Can you work these out from the model? Positions are in its coordinate system, mm. Face numbers are marked on the shaded views. Round coordinates to 2 decimals unless told otherwise and drop trailing zeros. Loops run counter-clockwise (first coordinate to the right, second up) from the corner with the lowest first, then second, coordinate; pieces in that order, holes last.
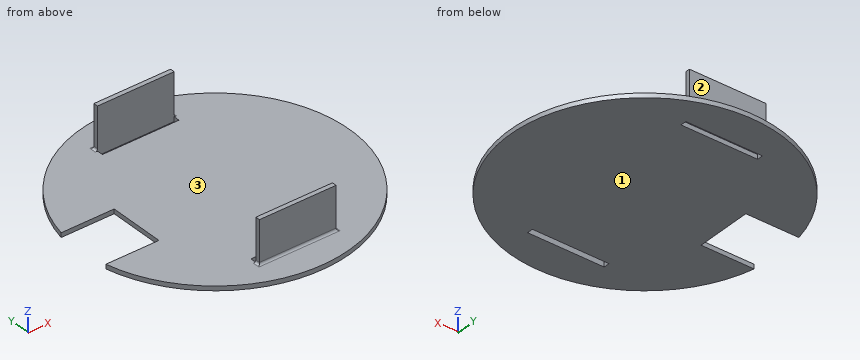
```python
from build123d import *

# Parameters (mm, degrees)
CROQUIS1_W              = 34.2
CROQUIS1_H              = 2.7
SALIENTE_EXTRUIR1_DEPTH = 2
CROQUIS2_W              = 34.2
CROQUIS2_H              = 2
SALIENTE_EXTRUIR2_DEPTH = 19
REDONDEO1_R             = 1


with BuildPart() as part:
    # Croquis1 → Saliente-Extruir1 (new body)
    with BuildSketch(Plane.XY):
        with BuildLine():
            Line((-58.683472972, -12.5), (-35, -12.5))
            Line((-35, -12.5), (-35, 12.5))
            Line((-35, 12.5), (-58.683472972, 12.5))
            ThreePointArc((-58.683472972, 12.5), (60, 0), (-58.683472972, -12.5))
        make_face()
        with Locations((0, 42.85)):
            Rectangle(CROQUIS1_W, CROQUIS1_H, mode=Mode.SUBTRACT)
        with Locations((0, -42.85)):
            Rectangle(CROQUIS1_W, CROQUIS1_H, mode=Mode.SUBTRACT)
    extrude(amount=SALIENTE_EXTRUIR1_DEPTH)

    # Croquis2 → Saliente-Extruir2 (add)
    with BuildSketch(Plane.XY.offset(2)):
        with Locations((0, 45.2)):
            Rectangle(CROQUIS2_W, CROQUIS2_H)
        with Locations((0, -45.2)):
            Rectangle(CROQUIS2_W, CROQUIS2_H)
    extrude(amount=SALIENTE_EXTRUIR2_DEPTH)

    # Redondeo1
    redondeo1_edges = [part.edges().sort_by_distance(p)[0] for p in [
        (-17.1, 45.2, 2),
        (17.1, 45.2, 2),
        (0, 46.2, 2),
        (-17.1, -45.2, 2),
        (0, -46.2, 2),
        (17.1, -45.2, 2),
    ]]
    fillet(redondeo1_edges, radius=REDONDEO1_R)


solid = part.part
```
(1) We'd pull the mould along Y, two halves only. Please class the marked faces 1, 2 and 3: released by +Y, released by -Y, zero draft, split by the parting line, or undercut.
(2) For pin 1 (1 mm diameter, centred on y = 42, z = 1, fed in from +X); pin 2 (1 mm diameter, centred on y = 45, z = 8, fed in from +X); pin 3 (2 mm diameter, centred on x = -41, z = 1.5, fed in from -Y); pin 4 (12 mm diameter, centred on x = -41, z = 9.5, fed in from +Y), each with a flat end and sliding along its axis, tell me the tip position at first contact or that it passes through.
(3) If I drill on line 1 (Y direction, x = -13, z = 6.75); line 2 (Z direction, x = 4.5, y = 38.5); line 3 (X direction, y = 46, z = 11.25), over which ranges is the centre line in solid material (lowest first)?
(4) Suppose I cut it at C-C (x = -43.5). Write out the boundary of the cut face in (y, z), then the cut area to 3 significant figures.
(5) Suppose I cut it at D-D (y = 0). Write out the boundary of the cut face in (x, z), then the cut area to 3 significant figures.
(6) Suppose I cut it at A-A (z = 18.75). Write out the boundary of the cut face in (x, y), then the cut area to 3 significant figures.
(7) Suppose I cut it at B-B (x = 0). Write out the boundary of the cut face in (y, z).
Check result:
1. face 1: zero draft
1. face 2: released by +Y
1. face 3: undercut
2. pin 1: stops at x = 43.33
2. pin 2: stops at x = 17.1
2. pin 3: stops at y = -44.72
2. pin 4: passes through
3. line 1: y = -46.2 to -44.2, 44.2 to 46.2
3. line 2: z = 0 to 2
3. line 3: x = -17.1 to 17.1
4. outline: (-41.32, 0) - (-12.5, 0) - (-12.5, 2) - (-41.32, 2) - close; (12.5, 0) - (41.32, 0) - (41.32, 2) - (12.5, 2) - close
4. area: 115 mm2
5. outline: (-35, 0) - (60, 0) - (60, 2) - (-35, 2) - close
5. area: 190 mm2
6. outline: (-17.1, -46.2) - (17.1, -46.2) - (17.1, -44.2) - (-17.1, -44.2) - close; (-17.1, 44.2) - (17.1, 44.2) - (17.1, 46.2) - (-17.1, 46.2) - close
6. area: 137 mm2
7. outline: (-60, 0) - (-44.2, 0) - (-44.2, 21) - (-46.2, 21) - (-46.2, 3) arc R1 cw to (-47.2, 2) - (-60, 2) - close; (-41.5, 0) - (41.5, 0) - (41.5, 2) - (-41.5, 2) - close; (44.2, 0) - (60, 0) - (60, 2) - (47.2, 2) arc R1 cw to (46.2, 3) - (46.2, 21) - (44.2, 21) - close
